Design review of the part built by this model. Coordinates are the model's own, in mm. A direction names the side the tool comes from. Round coordinates to 2 decimals unless told otherwise and drop trailing zeros. Write each loop counter-clockwise with the first axis right and the second up, starting at its lowest first coordinate (ties: lowest second). Pieces come first, ordered by that corner, then holes.
from build123d import *

# Parameters (mm, degrees)
CHAMFER_1_SIZE = 1
CHAMFER_2_SIZE = 1


with BuildPart() as part:
    # 草图1 → 旋转1 (revolve)
    with BuildSketch(Plane.XY, mode=Mode.PRIVATE) as revolve_1_sk:
        with BuildLine():
            Line((0, 0), (0, 7))
            ThreePointArc((0, 7), (0.292893219, 7.707106781), (1, 8))
            Line((1, 8), (11, 8))
            Line((11, 8), (11, 10))
            Line((11, 10), (21, 10))
            Line((21, 10), (21, 8))
            Line((21, 8), (30, 8))
            Line((30, 8), (30, 5))
            Line((30, 5), (32, 5))
            Line((32, 5), (32, 6))
            Line((32, 6), (40, 6))
            Line((40, 6), (40, 0))
            Line((40, 0), (0, 0))
        make_face()
    revolve(revolve_1_sk.sketch.rotate(Axis((0, 0, 0), (1, 0, 0)), 90), axis=Axis((0, 0, 0), (1, 0, 0)))

    # 倒角1
    chamfer_1_edges = [part.edges().sort_by_distance(p)[0] for p in [
        (11, 0, -10),
        (21, 0, -10),
    ]]
    chamfer(chamfer_1_edges, length=CHAMFER_1_SIZE)

    # 倒角2
    chamfer_2_edges = [part.edges().sort_by_distance(p)[0] for p in [
        (40, 0, -6),
    ]]
    chamfer(chamfer_2_edges, length=CHAMFER_2_SIZE)


solid = part.part
1) Add section A-A on y = 0. State the section outline as (x, z) points, and give its area (3 significant figures).
2) Add section C-C on x = 13.5. State the section outline as (y, z) points, and give its area (3 significant figures).
3) For line 1 along X through (y, z) = (4.75, 4.25); line 2 along Y through (x, z) = (29.5, 6.25); line 3 along X through (y, z) = (-1.25, 5.5), list the stretches that pass through material, from the lowest coordinate up.
4) For faces 1 (the face through (16, 0, -10)), 2 (the face through (0, 0, 0)), 3 (the face through (6.07, 7.81, -1.73)), 4 (the face through (31, 0, -5)), 5 (the face through (35.549, -1.802, 5.723)), list the 3-axis set-ups (+Z, -Z, +X, -X, +Y, -Y) from which the entire face can be reached by the end or side of a thin tool; tool diameter is ignored.
5) For P1, Ø5, axis at x = 5, z = -3, coming from the +Y side; P2, Ø12, axis at x = 32, y = -2, coming from the +Z side; P3, Ø1.5, axis at y = 3.5, z = -4.5, coming from the +X side; P4, Ø4, axis at x = 34.5, y = -5.5, coming from the -Z side, all flat-tipped, find the tip position at first contact; note any pin that passes through.
6) Add section D-D on x = 29. State the section outline as (y, z) points.
Computed:
1. outline: (0, -7) arc R1 ccw to (1, -8) - (11, -8) - (11, -9) - (12, -10) - (20, -10) - (21, -9) - (21, -8) - (30, -8) - (30, -5) - (32, -5) - (32, -6) - (39, -6) - (40, -5) - (40, 5) - (39, 6) - (32, 6) - (32, 5) - (30, 5) - (30, 8) - (21, 8) - (21, 9) - (20, 10) - (12, 10) - (11, 9) - (11, 8) - (1, 8) arc R1 ccw to (0, 7) - close
1. area: 633 mm2
2. outline: circle Ø20 at (0, 0)
2. area: 314 mm2
3. line 1: x = 0 to 30
3. line 2: y = -4.99 to 4.99
3. line 3: x = 0 to 30, 32 to 39.36
4. face 1: +X, -X
4. face 2: +Z, -Z, -X, +Y, -Y
4. face 3: -X
4. face 4: none
4. face 5: +X
5. P1: stops at y = 7.98
5. P2: stops at z = 8
5. P3: stops at x = 40
5. P4: stops at z = -4.87
6. outline: circle Ø16 at (0, 0)
